Autodesk Inventor part; units mm, degrees
ref_plane "YZ Plane" through (0, 0, 0) normal (1, 0, 0) x (0, 1, 0)
ref_plane "XZ Plane" through (0, 0, 0) normal (0, 1, 0) x (-1, 0, 0)
ref_plane "XY Plane" through (0, 0, 0) normal (0, 0, 1) x (1, 0, 0)
sketch "Sketch1" plane through (0, 0, 0) normal (0, 1, 0) x (-1, 0, 0)
  line L0 (-9, 6) -> (-9, -6)
  line L1 (-9, -6) -> (9, -6)
  line L2 (9, -6) -> (9, 6)
  line L3 (9, 6) -> (-9, 6)
  line L4 (-9, 6) -> (9, -6) construction
  line L5 (-9, -6) -> (9, 6) construction
  point P0 (0, 0)
  dimension "d0" = 12
  dimension "d1" = 18
extrude "Extrusion1" add sketch "Sketch1" along normal blind 12
sketch "Sketch2" plane through (0, 12, 0) normal (0, 1, 0) x (1, 0, 0)
  line L0 (10.5, -7.5) -> (10.5, 7.5)
  line L1 (10.5, 7.5) -> (-10.5, 7.5)
  line L2 (-10.5, 7.5) -> (-10.5, -7.5)
  line L3 (-10.5, -7.5) -> (10.5, -7.5)
  line L4 (10.5, -7.5) -> (-10.5, 7.5) construction
  line L5 (10.5, 7.5) -> (-10.5, -7.5) construction
  point P0 (0, 0)
  dimension "d4" = 15
  dimension "d5" = 21
extrude "Extrusion2" add sketch "Sketch2" along normal blind 2
chamfer "Chamfer1" distance 1.8 distance2 1.2 1 edges at (10.5, 14, 0) measured on face at (3.5, 14, 2.5)
chamfer "Chamfer2" distance 1.8 distance2 1.2 1 edges at (-0.9, 14, 7.5) measured on face at (2.3, 14, 2.5)
chamfer "Chamfer3" distance 1.8 distance2 1.2 1 edges at (-10.5, 14, -0.9) measured on face at (-4.1, 14, 1.3)
chamfer "Chamfer4" distance 1.8 distance2 1.2 1 edges at (0, 14, -7.5) measured on face at (2.9, 14, 1.3)
sketch "Sketch3" plane through (0, 14, 0) normal (0, 1, 0) x (1, 0, 0)
  line L0 (-8.7, 5.7) -> (8.7, 5.7)
  line L1 (-8.7, -5.7) -> (-8.7, 5.7)
  line L2 (8.7, -5.7) -> (-8.7, -5.7)
  line L3 (8.7, 5.7) -> (8.7, -5.7)
  point P0 (0, 0)
extrude "Extrusion3" add sketch "Sketch3" along normal blind 3
sketch "Sketch4" plane through (-8.7, 14, 5.7) normal (0, 0, 1) x (1, 0, 0)
  line L0 (17.4, 0) -> (0, 0)
  line L1 (17.4, 0) -> (17.4, 3)
  line L2 (0, 3) -> (17.4, 3)
  line L3 (0, 0) -> (0, 3)
  line L4 (17.4, 0) -> (17.4, 3)
  line L5 (17.4, 3) -> (0, 3)
  line L6 (0, 3) -> (0, 0)
  line L7 (0, 0) -> (17.4, 0)
  line L8 (17.4, 0) -> (16.7, 0)
  line L9 (17.4, 0) -> (0, 0)
  line L10 (16.7, 0) -> (16.7, 3)
  line L11 (0, 3) -> (17.4, 3)
  arc A0 (0, 0) -> (16.7, 3) centre (-4.649, 73.861) ccw
  arc A1 (17.4, 0) -> (16.7, 3) centre (10.8425, 0.0516) ccw
  point P0 (8.7, -14)
  dimension "d24" = 0.7
extrude "Extrusion4" cut sketch "Sketch4" against normal through all contours A1 L2 L1 | A0 L3 L2
sketch "Sketch5" plane through (0, 0, 0) normal (0, -1, 0) x (1, 0, 0)
  line L0 (0.5, -4) -> (0.5, 4)
  line L1 (0.5, 4) -> (-0.5, 4)
  line L2 (-0.5, 4) -> (-0.5, -4)
  line L3 (-0.5, -4) -> (0.5, -4)
  line L4 (0.5, -4) -> (-0.5, 4) construction
  line L5 (0.5, 4) -> (-0.5, -4) construction
  line L6 (0, 0) -> (-6, 0)
  line L7 (0, 0) -> (6, 0)
  line L8 (-5.5, -4) -> (-5.5, 4)
  line L9 (-5.5, 4) -> (-6.5, 4)
  line L10 (-6.5, 4) -> (-6.5, -4)
  line L11 (-6.5, -4) -> (-5.5, -4)
  line L12 (-5.5, -4) -> (-6.5, 4) construction
  line L13 (-5.5, 4) -> (-6.5, -4) construction
  line L14 (6.5, -4) -> (6.5, 4)
  line L15 (6.5, 4) -> (5.5, 4)
  line L16 (5.5, 4) -> (5.5, -4)
  line L17 (5.5, -4) -> (6.5, -4)
  line L18 (6.5, -4) -> (5.5, 4) construction
  line L19 (6.5, 4) -> (5.5, -4) construction
  dimension "d27" = 8
  dimension "d28" = 1
  dimension "d29" = 6
  dimension "d30" = 6
  dimension "d31" = 1
  dimension "d32" = 1
extrude "Extrusion5" add sketch "Sketch5" along normal blind 8
chamfer "Chamfer5" distance 2 angle 45 6 edges at (6, -8, -4) (6, -8, 4) (0, -8, 4) (-6, -8, 4) (-6, -8, -4) (0, -8, -4)
sketch "Sketch6" plane through (-6.5, 0, -4) normal (-1, 0, 0) x (0, 0, 1)
  circle A0 centre (4, -5.0131) radius 1.5
  point P0 (4, 0)
  dimension "d38" = 3
extrude "Extrusion6" cut sketch "Sketch6" against normal blind 24.25
properties part number "Toggle switch"
CAD build for the part. Positions are in the model's coordinates, mm. A direction names the side the tool comes from. Give positions to 0.01 mm unless a question says otherwise; leave off trailing zeros. Write each loop counter-clockwise with the first axis right and the second up, starting at its lowest first coordinate (ties: lowest second). Pieces come first, ordered by that corner, then holes. Notation, with made-up numbers: (-2, 53) -> (25, 53) arc R15 ccw to (25, 66) -> close; hole circle Ø10 at (-6.5, -3). An arc over 180 degrees is marked (long way). Return JSON: item names as keys, results as strings.
Item 1: Drill centre lines: probe 1 along X at (y, z) = (-6, -3.25); probe 2 along Z at (x, y) = (2.75, 9.5); probe 3 along Y at (x, z) = (-0.3, 0). Where is each one in solid material? Low to high.
Answer below:
{"probe 1": "x = -6.5 to -5.5, -0.5 to 0.5, 5.5 to 6.5", "probe 2": "z = -6 to 6", "probe 3": "y = -8 to -6.51, -3.51 to 15.01"}
Item 2: Band-saw the part on A-A (y = -1.75). List the corners of the cut face in (x, z).
Answer below:
{"outline": "(-6.5, -4) -> (-5.5, -4) -> (-5.5, 4) -> (-6.5, 4) -> close; (-0.5, -4) -> (0.5, -4) -> (0.5, 4) -> (-0.5, 4) -> close; (5.5, -4) -> (6.5, -4) -> (6.5, 4) -> (5.5, 4) -> close"}
Item 3: Tool access for faces 5 (the flat face through (4, 15, 5.7)), 6 (the flat face through (0, 12, 7)), 7 (the flat face through (-6, -3, -4)), 8 (the flat face through (-6, -3, 4)): list every direction of +Z, -Z, +X, -X, +Y, -Y with a clear straight run to the whole face (end or side of a thin tool).
Answer below:
{"face 5": "+Z, +X, -X, +Y", "face 6": "-Y", "face 7": "-Z, +X, -X, -Y", "face 8": "+Z, +X, -X, -Y"}
Item 4: Drop flat-ended pins along their axis: pin 1 (2.5 mm diameter, centred on x = 3, y = 15.5, fed in from -Z); pin 2 (3 mm diameter, centred on x = 5.5, y = 6, fed in from -Z); pin 3 (6 mm diameter, centred on x = 6, y = 0.5, fed in from +Z). Give the stop position or say it passes through.
Answer below:
{"pin 1": "stops at z = -5.7", "pin 2": "stops at z = -6", "pin 3": "stops at z = 6"}
Item 5: Band-saw the part on D-D (z = 0). Give the number of separate pieces and of enclosed holes in the cut face, then the cut area to 3 significant figures.
Answer below:
{"separate pieces": "4", "enclosed holes": "0", "area": "292 mm2"}
Item 6: Band-saw the part on B-B (z = -5). List the corners of the cut face in (x, y).
Answer below:
{"outline": "(-10.5, 12) -> (-9, 12) -> (-9, 0) -> (9, 0) -> (9, 12) -> (10.5, 12) -> (10.5, 12.8) -> (8.7, 14) arc R6.56 ccw to (8, 17) arc R74.01 cw to (-8.7, 14) -> (-10.5, 12.8) -> close"}
Item 7: Two-plate mould, pull along X, no slides. Class faces 1 (the cylindrical face through (-0.38, 15, 0.08)), 2 (the flat face through (9.6, 13.4, 0.1)), 3 (the flat face through (-6, -7, -3)), 4 (the flat face through (5.5, -3, 0)): +X half, -X half, draft (parallel to the pull), parting line (faces both ways), or undercut.
Answer below:
{"face 1": "-X half", "face 2": "+X half", "face 3": "draft", "face 4": "undercut"}
Item 8: Band-saw the part on C-C (x = 3.5). List the corners of the cut face in (y, z).
Answer below:
{"outline": "(0, -6) -> (12, -6) -> (12, -7.5) -> (12.8, -7.5) -> (14, -5.7) -> (15.8, -5.7) -> (15.8, 5.7) -> (14, 5.7) -> (12.8, 7.5) -> (12, 7.5) -> (12, 6) -> (0, 6) -> close"}
